CAD build for the part. Positions are in the model's coordinates, mm. A direction names the side the tool comes from. Give positions to 0.01 mm unless a question says otherwise; leave off trailing zeros. Answer as a JSON object with one key per item and string values.
Autodesk Inventor part; units mm, degrees
ref_plane "YZ Plane" through (0, 0, 0) normal (1, 0, 0) x (0, 1, 0)
ref_plane "XZ Plane" through (0, 0, 0) normal (0, 1, 0) x (-1, 0, 0)
ref_plane "XY Plane" through (0, 0, 0) normal (0, 0, 1) x (1, 0, 0)
sketch "Sketch1" plane through (0, 0, 0) normal (0, 0, 1) x (1, 0, 0)
  line L0 (-2.205, 0) -> (2.205, 0)
  line L1 (0, -2.205) -> (0, 2.205)
  arc A0 (9, -10) -> (10, -9) centre (9, -9) ccw
  line L2 (-10, 9) -> (-10, 3)
  line L3 (-10, 3) -> (-8, 3)
  line L4 (-8, 3) -> (-8, 6)
  line L5 (-8, 6) -> (-7.0607, 6)
  line L6 (-7.0607, 6) -> (-4, 2.9393)
  line L7 (-4, 2.9393) -> (-4, 0.5196)
  line L8 (-4, 0.5196) -> (-3.7, 0)
  line L9 (-3.7, 0) -> (-4, -0.5196)
  line L10 (-4, -0.5196) -> (-4, -2.9393)
  line L11 (-4, -2.9393) -> (-7.0607, -6)
  line L12 (-7.0607, -6) -> (-8, -6)
  line L13 (-8, -6) -> (-8, -3)
  line L14 (-8, -3) -> (-10, -3)
  line L15 (-10, -3) -> (-10, -9)
  arc A1 (-10, -9) -> (-9, -10) centre (-9, -9) ccw
  line L16 (-9, -10) -> (-3, -10)
  line L17 (-3, -10) -> (-3, -8)
  line L18 (-3, -8) -> (-6, -8)
  line L19 (-6, -7.0607) -> (-2.9393, -4)
  line L20 (-2.9393, -4) -> (-0.5196, -4)
  line L21 (-0.5196, -4) -> (0, -3.7)
  line L22 (0, -3.7) -> (0.5196, -4)
  line L23 (0.5196, -4) -> (2.9393, -4)
  line L24 (2.9393, -4) -> (6, -7.0607)
  line L25 (6, -7.0607) -> (6, -8)
  line L26 (6, -8) -> (3, -8)
  line L27 (3, -8) -> (3, -10)
  line L28 (3, -10) -> (9, -10)
  line L29 (10, -9) -> (10, -3)
  line L30 (10, -3) -> (8, -3)
  line L31 (8, -3) -> (8, -6)
  line L32 (8, -6) -> (7.0607, -6)
  line L33 (7.0607, -6) -> (4, -2.9393)
  line L34 (4, -2.9393) -> (4, -0.5196)
  line L35 (4, -0.5196) -> (3.7, 0)
  line L36 (3.7, 0) -> (4, 0.5196)
  line L37 (4, 0.5196) -> (4, 2.9393)
  line L38 (4, 2.9393) -> (7.0607, 6)
  line L39 (7.0607, 6) -> (8, 6)
  line L40 (8, 6) -> (8, 3)
  line L41 (8, 3) -> (10, 3)
  line L42 (10, 3) -> (10, 9)
  arc A2 (10, 9) -> (9, 10) centre (9, 9) ccw
  line L43 (9, 10) -> (3, 10)
  line L44 (3, 10) -> (3, 8)
  line L45 (3, 8) -> (6, 8)
  line L46 (6, 8) -> (6, 7.0607)
  line L47 (6, 7.0607) -> (2.9393, 4)
  line L48 (2.9393, 4) -> (0.5196, 4)
  line L49 (0.5196, 4) -> (0, 3.7)
  line L50 (0, 3.7) -> (-0.5196, 4)
  line L51 (-0.5196, 4) -> (-2.9393, 4)
  line L52 (-2.9393, 4) -> (-6, 7.0607)
  line L53 (-6, 7.0607) -> (-6, 8)
  line L54 (-6, 8) -> (-3, 8)
  line L55 (-3, 8) -> (-3, 10)
  line L56 (-3, 10) -> (-9, 10)
  arc A3 (-9, 10) -> (-10, 9) centre (-9, 9) ccw
  circle A4 centre (0, 0) radius 2.1
  line L57 (-6, -8) -> (-6, -7.0607)
extrude "Extrusion1" add sketch "Sketch1" along normal mid plane 200
properties part number "15 cm extrusion" material "Aluminum 6061"
1) 3-axis set-ups, long thin cutter, end or side, ignore diameter. For faces 5 (the flat face through (-0.1, 2.4, 100)), 6 (the flat face through (5.55, -4.49, -1.4)): which of +Z, -Z, +X, -X, +Y, -Y reach the whole face in a straight line?
Model answer:
{"face 5": "+Z, +X, -X, +Y, -Y", "face 6": "+Z, -Z"}
2) Pin check, flat tips, straight feed: pin 1 (1 mm diameter, centred on x = 1, z = 15, fed in from +Y); pin 2 (1.9 mm diameter, centred on x = -1, z = 25.5, fed in from -Y); pin 3 (0.7 mm diameter, centred on y = 2, z = 26.5, fed in from +X); pin 4 (2.5 mm diameter, centred on x = 0, y = 0, fed in from +Z). Stop position of each tip, or through.
Model answer:
{"pin 1": "stops at y = 4", "pin 2": "stops at y = -4", "pin 3": "stops at x = 4", "pin 4": "passes through"}
3) Wall check: probe 1 along X at (y, z) = (0, 3.5); probe 2 along Y at (x, z) = (7.75, 21). Give the ranges that are in metal, low to high.
Model answer:
{"probe 1": "x = -3.7 to -2.1, 2.1 to 3.7", "probe 2": "y = -10 to -6, 6 to 10"}
4) Mould opens along X. For faces 1 (the flat face through (-10, -6, -1)), 2 (the flat face through (6, -10, -1)), 3 (the flat face through (10, -6, -1)), 4 (the flat face through (-5.51, -4.45, -1.4)) say: released by +X, released by -X, zero draft, split by the parting line, or undercut.
Model answer:
{"face 1": "released by -X", "face 2": "zero draft", "face 3": "released by +X", "face 4": "undercut"}
